from build123d import *

# Parameters (mm, degrees)
BOSS_EXTRUDE1_DEPTH     = 24
SKETCH2_R               = 2
CUT_EXTRUDE1_DEPTH      = 24
SKETCH3_R               = 3
CUT_EXTRUDE2_DEPTH      = 1
CUT_EXTRUDE2_DEPTH_BACK = 37
SKETCH4_W               = 3.175
SKETCH4_H               = 24
BOSS_EXTRUDE2_DEPTH     = 101.6
SKETCH7_R               = 2.032
CUT_EXTRUDE3_DEPTH      = 4.175
FILLET1_R               = 5
FILLET2_R               = 5


with BuildPart() as part:
    # Sketch1 → Boss-Extrude1 (new body)
    with BuildSketch(Plane(origin=(0, 0, 0), x_dir=(1, 0, 0), z_dir=(0, 1, 0))):
        Polygon((12.5, -16.134036145), (12.5, 16.365963855), (-12.5, 16.365963855), (-12.5, -16.134036145), (-18, -16.134036145), (-18, 22.365963855), (18, 22.365963855), (18, -16.134036145), align=None)
    extrude(amount=BOSS_EXTRUDE1_DEPTH)

    # Sketch2 → Cut-Extrude1 (cut)
    with BuildSketch(Plane(origin=(0, 0, -22.365963855), x_dir=(-1, 0, 0), z_dir=(0, 0, -1))):
        with Locations((0, 12)):
            Circle(SKETCH2_R)
    extrude(amount=-CUT_EXTRUDE1_DEPTH, mode=Mode.SUBTRACT)

    # Sketch3 → Cut-Extrude2 (cut, two sides)
    with BuildSketch(Plane.ZY.offset(18)) as cut_extrude2_sk:
        with Locations((3.634036145, 12)):
            Circle(SKETCH3_R)
    extrude(amount=CUT_EXTRUDE2_DEPTH, mode=Mode.SUBTRACT)
    extrude(cut_extrude2_sk.sketch, amount=-CUT_EXTRUDE2_DEPTH_BACK, mode=Mode.SUBTRACT)

    # Sketch4 → Boss-Extrude2 (add)
    with BuildSketch(Plane.ZY.offset(18)):
        with Locations((14.546536145, 12)):
            Rectangle(SKETCH4_W, SKETCH4_H)
    boss_extrude2 = extrude(amount=BOSS_EXTRUDE2_DEPTH)

    # Sketch7 → Cut-Extrude3 (cut, through all)
    with BuildSketch(Plane(origin=(0, 0, 12.959036145), x_dir=(-1, 0, 0), z_dir=(0, 0, -1))):
        with Locations((30, 12)):
            Circle(SKETCH7_R)
        with Locations((55, 12)):
            Circle(SKETCH7_R)
        with Locations((80, 12)):
            Circle(SKETCH7_R)
        with Locations((105, 12)):
            Circle(SKETCH7_R)
        with Locations((130, 12)):
            Circle(SKETCH7_R)
        with Locations((155, 12)):
            Circle(SKETCH7_R)
    cut_extrude3 = extrude(amount=-CUT_EXTRUDE3_DEPTH, mode=Mode.SUBTRACT)

    # Mirror1: Boss-Extrude2, Cut-Extrude3 across plane
    add(boss_extrude2.mirror(Plane.ZY))
    add(cut_extrude3.mirror(Plane.ZY), mode=Mode.SUBTRACT)

    # Fillet1
    fillet1_edges = [part.edges().sort_by_distance(p)[0] for p in [
        (-18, 12, 12.959036145),
    ]]
    fillet(fillet1_edges, radius=FILLET1_R)

    # Fillet2
    fillet2_edges = [part.edges().sort_by_distance(p)[0] for p in [
        (18, 12, 12.959036145),
    ]]
    fillet(fillet2_edges, radius=FILLET2_R)


solid = part.part
Could you check a few things on this model? Use its own coordinates, in mm. A direction names the side the tool comes from. Round coordinates to 2 decimals unless told otherwise and drop trailing zeros. Order: outer loops, then holes, each group sorted by start corner. A loop starts at its lowest first (then second) coordinate and runs counter-clockwise, first axis right, second up. Notation, with made-up numbers: M 69,-19.75 L 107,-19.75 A20 cw 107,-12.75 Z; hole C -30.5,2.5 d1. An arc over 180 degrees is marked long. One line per item, written item: value.
(1) If we mould it in two halves opening along Y, with no side actions, what happens to faces 1 (the flat face through (-12.5, 12, 0)), 2 (the flat face through (17, 0, 4)), 3 (the cylindrical face through (52.97, 12.09, 14.52)), 4 (the cylindrical face through (-15.288, 10.851, 6.405))? For each: released by +Y, released by -Y, zero draft, split by the parting line, or undercut.
Ans:
face 1: zero draft
face 2: released by -Y
face 3: undercut
face 4: undercut
(2) Imagine slicing it at D-D (x = -15). Write out the boundary of the cut face in (y, z), and give its area (3 significant figures).
Ans:
outline: M 0,-22.37 L 24,-22.37 L 24,16.13 L 0,16.13 Z; hole C 12,3.63 d6
area: 896 mm^2
(3) Imagine slicing it at A-A (z = -11). Write out the boundary of the cut face in (x, y), and give its area (3 significant figures).
Ans:
outline: M -18,0 L -12.5,0 L -12.5,24 L -18,24 Z; M 12.5,0 L 18,0 L 18,24 L 12.5,24 Z
area: 264 mm^2
(4) Imagine slicing it at C-C (y = 17.5). Write out the boundary of the cut face in (x, z).
Ans:
outline: M -119.6,12.96 L -23,12.96 A5 cw -18,7.96 L -18,-22.37 L 18,-22.37 L 18,7.96 A5 cw 23,12.96 L 119.6,12.96 L 119.6,16.13 L 12.5,16.13 L 12.5,-16.37 L -12.5,-16.37 L -12.5,16.13 L -119.6,16.13 Z
(5) I need wall thicknesses on line 1 along X through (y, z) = (13.25, -4); line 2 along Y through (x, z) = (0, -18); line 3 along Z through (x, y) = (40, 21.5). Which ranges of each line are inside material? Lowest first, please. Write a range as from..to.
Ans:
line 1: x = -18..-12.5, 12.5..18
line 2: y = 0..10, 14..24
line 3: z = 12.96..16.13
(6) Which directions (+Z, -Z, +X, -X, +Y, -Y) give clear straight access to the entire face, cutting with the end or side of a thin tool? Please do faces 5 (the cylindrical face through (-52.97, 12.09, 14.52)), 6 (the flat face through (18, 12, -7)), 7 (the flat face through (-65, 12, 16.134)), 8 (the flat face through (-71, 12, 12.959)), 9 (the flat face through (12.5, 12, 0)).
Ans:
face 5: +Z, -Z
face 6: -Z, +X, +Y, -Y
face 7: +Z, +X, -X, +Y, -Y
face 8: -Z, -X, +Y, -Y
face 9: +Z, +Y, -Y
(7) Imagine slicing it at B-B (x = -55). Write out the boundary of the cut face in (y, z).
Ans:
outline: M 0,12.96 L 9.97,12.96 L 9.97,16.13 L 0,16.13 Z; M 14.03,12.96 L 24,12.96 L 24,16.13 L 14.03,16.13 Z
(8) I'm going to push flat-ended pins straight in: P1, Ø1.5, axis at x = -16, z = 12, coming from the -Y side; P2, Ø12, axis at y = 17.5, z = -14.5, coming from the +X side; P3, Ø7, axis at x = 1.5, y = 16.5, coming from the +Z side; P4, Ø7, axis at x = -91, y = 15, coming from the -Z side. Where does each tip first touch, or does it pass through?
Ans:
P1: stops at y = 0
P2: stops at x = 18
P3: stops at z = -16.37
P4: stops at z = 12.96
